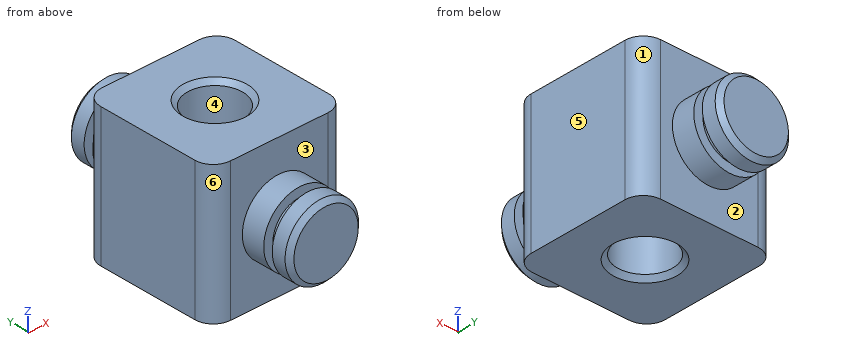
```python
from build123d import *

# Parameters (mm, degrees)
F0_R     = 3
F1_DEPTH = 7.5
F2_SIZE2 = 0.5
F2_SIZE  = 0.5
F3_R     = 4
F4_DEPTH = 5.5
F5_SIZE2 = 0.5
F5_SIZE  = 0.5
F6_W     = 1
F6_H     = 1


# Not quite as in the source:
# - a feature of the source that left no trace in its solid (it failed there, or was rolled back) is left out
# - a pattern or mirror of a feature is missing from the dataset's text; its kind, count and spacing are read off the source's solid


with BuildPart() as f1:
    # F0 (on Top) → F1 (new body, symmetric)
    with BuildSketch(Plane.XY):
        with BuildLine():
            ThreePointArc((7.3, 5.5), (6.7142135624, 6.9142135624), (5.3, 7.5))
            Line((5.3, 7.5), (-5.3, 7.5))
            ThreePointArc((-5.3, 7.5), (-6.7142135624, 6.9142135624), (-7.3, 5.5))
            Line((-7.3, 5.5), (-7.3, -5.5))
            ThreePointArc((-7.3, -5.5), (-6.7142135624, -6.9142135624), (-5.3, -7.5))
            Line((-5.3, -7.5), (5.3, -7.5))
            ThreePointArc((5.3, -7.5), (6.7142135624, -6.9142135624), (7.3, -5.5))
            Line((7.3, -5.5), (7.3, 5.5))
        make_face()
        Circle(F0_R, mode=Mode.SUBTRACT)
    extrude(amount=F1_DEPTH, both=True)

    # F2
    f2_edges = [f1.edges().sort_by_distance(p)[0] for p in [
        (-3, 0, 7.5),
        (-3, 0, -7.5),
    ]]
    chamfer(f2_edges, length=F2_SIZE, length2=F2_SIZE2)

    # F3 (on face) → F4 (join)
    with BuildSketch(Plane.XZ.offset(7.5)):
        Circle(F3_R)
    f4 = extrude(amount=F4_DEPTH)

    # F4_copies: F4 across plane
    add(f4.mirror(Plane.ZX))

    # F5
    f5_edges = [f1.edges().sort_by_distance(p)[0] for p in [
        (-4, -13, 0),
        (-4, 13, 0),
    ]]
    chamfer(f5_edges, length=F5_SIZE, length2=F5_SIZE2)

    # F6 (on Right) → F7 (revolve, cut)
    with BuildSketch(Plane.YZ):
        with Locations((-10.5, 3.5)):
            Rectangle(F6_W, F6_H)
    f7 = revolve(axis=Axis((0, -13, 0), (0, -1, 0)), mode=Mode.SUBTRACT)

    # F7_copies: F7 across plane
    add(f7.mirror(Plane.ZX), mode=Mode.SUBTRACT)


solid = f1.part
```
Design review of the part built by this model. Coordinates are the model's own, in mm. Face numbers are marked on the shaded views. A direction names the side the tool comes from. Coordinates: 2 decimals unless noted, no trailing zeros. Write each loop counter-clockwise with the first axis right and the second up, starting at its lowest first coordinate (ties: lowest second). Pieces come first, ordered by that corner, then holes.
1) Add section A-A (y = 0). Write out the cut boundary in (x, z), plus the area to 4 significant figures.
2) Add section B-B (x = -5.75). Write out the cut boundary in (y, z), plus the area to 3 significant figures.
3) Add section C-C (y = -7). Write out the cut boundary in (x, z).
4) Insertion check: pin 1 (4 mm diameter, centred on x = -2.5, z = -5.5, fed in from +Y). The pin has a flat end and moves straight along its axis. Give the tip position at first contact, or say it passes through.
5) Machinability: for the marked faces 1, 2 and 3, which of the approach directions +Z, -Z, +X, -X, +Y, -Y give a long, thin tool a straight path to every point of the face, cutting with its end or side? Answer none if there is none.
6) To check wall thickness, follow L1, parallel to Y at x = -1.5, z = -2.75; L2, parallel to Y at x = 0, z = -1.25; L3, parallel to Y at x = -2, z = 2.75. State the ranges of each line that lie inside material, in increasing order.
7) Mouldability with a two-part tool opening along Y and no side actions: class the marked faces 4, 5 and 6 as +Y half, -Y half, draft (parallel to the pull), parting line (faces both ways), or undercut.
Check result:
1. outline: (-7.3, -7.5) - (-3.5, -7.5) - (-3, -7) - (-3, 7) - (-3.5, 7.5) - (-7.3, 7.5) - close; (3, -7) - (3.5, -7.5) - (7.3, -7.5) - (7.3, 7.5) - (3.5, 7.5) - (3, 7) - close
1. area: 128.5 mm2
2. outline: (-7.45, -7.5) - (7.45, -7.5) - (7.45, 7.5) - (-7.45, 7.5) - close
2. area: 223 mm2
3. outline: (-6.62, -7.5) - (6.62, -7.5) - (6.62, 7.5) - (-6.62, 7.5) - close
4. pin 1: stops at y = 7.5
5. face 1: +Z, -Z, +X, +Y
5. face 2: +Y
5. face 3: -Y
6. L1: y = -13 to -11, -10 to -2.6, 2.6 to 10, 11 to 13
6. L2: y = -13 to -3, 3 to 13
6. L3: y = -13 to -11, -10 to -2.24, 2.24 to 10, 11 to 13
7. face 4: undercut
7. face 5: draft
7. face 6: -Y half
